```python
from build123d import *
from build123d.topology import SkipClean

# Parameters (mm, degrees)
SKETCH1_W           = 14
SKETCH1_H           = 42
BOSS_EXTRUDE1_DEPTH = 22.5
FILLET1_R           = 2
BOSS_EXTRUDE2_DEPTH = 18.5
BOSS_EXTRUDE3_DEPTH = 5
SKETCH4_R           = 1.1
CUT_EXTRUDE1_DEPTH  = 15
SKETCH5_W           = 2
SKETCH5_H           = 4
BOSS_EXTRUDE4_DEPTH = 5
BOSS_EXTRUDE5_DEPTH = 4
CUT_EXTRUDE2_START  = -2
CUT_EXTRUDE2_DEPTH  = 2
SKETCH12_R          = 3.5
SKETCH12_R_2        = 3.070336519
BOSS_EXTRUDE6_DEPTH = 1
SKETCH14_R          = 3
BOSS_EXTRUDE7_DEPTH = 1
SKETCH15_R          = 1
BOSS_EXTRUDE8_DEPTH = 7
SKETCH16_R          = 2
BOSS_EXTRUDE9_DEPTH = 1.5
CUT_EXTRUDE3_DEPTH  = 18.5


with BuildPart() as part:
    # Sketch1 → Boss-Extrude1 (new body)
    with BuildSketch(Plane(origin=(0, 0, 0), x_dir=(1, 0, 0), z_dir=(0, 1, 0))):
        with Locations((-14.72963025, -0.456790856)):
            Rectangle(SKETCH1_W, SKETCH1_H)
    extrude(amount=BOSS_EXTRUDE1_DEPTH)

    # Fillet1
    fillet1_edges = [part.edges().sort_by_distance(p)[0] for p in [
        (-14.72963025, 22.5, -20.543209144),
        (-14.72963025, 0, -20.543209144),
        (-14.72963025, 0, 21.456790856),
        (-14.72963025, 22.5, 21.456790856),
    ]]
    fillet(fillet1_edges, radius=FILLET1_R)

    # Sketch2 → Boss-Extrude2 (add)
    with BuildSketch(Plane(origin=(-7.72963025, 0, 0), x_dir=(0, 0, -1), z_dir=(1, 0, 0))):
        with BuildLine():
            Line((3.666133326, 18.67433994), (3.666133326, 3.82566006))
            ThreePointArc((3.666133326, 3.82566006), (12.136760187, 0.056811401), (20.543209144, 3.966716207))
            Line((20.543209144, 3.966716207), (20.543209144, 18.533283793))
            ThreePointArc((20.543209144, 18.533283793), (12.136760187, 22.443188599), (3.666133326, 18.67433994))
        make_face()
    extrude(amount=BOSS_EXTRUDE2_DEPTH)

    # Sketch3 → Boss-Extrude3 (add)
    with BuildSketch(Plane(origin=(-7.72963025, 0, 0), x_dir=(0, 0, -1), z_dir=(1, 0, 0))):
        with BuildLine():
            Line((3.666133326, 12.265446457), (3.666133326, 10.341158941))
            ThreePointArc((3.666133326, 10.341158941), (3.170141933, 10.546427574), (2.72390333, 10.248075799))
            ThreePointArc((2.72390333, 10.248075799), (-1.152649836, 11.204898318), (2.678489822, 12.329861741))
            ThreePointArc((2.678489822, 12.329861741), (3.155102255, 12.033793242), (3.666133326, 12.265446457))
        make_face()
    extrude(amount=BOSS_EXTRUDE3_DEPTH)

    # Sketch4 → Cut-Extrude1 (cut)
    with BuildSketch(Plane(origin=(-7.72963025, 0, 0), x_dir=(0, 0, -1), z_dir=(1, 0, 0))):
        with Locations((-18.956790856, 20)):
            Circle(SKETCH4_R)
        with Locations((-18.956790856, 2.5)):
            Circle(SKETCH4_R)
    extrude(amount=-CUT_EXTRUDE1_DEPTH, mode=Mode.SUBTRACT)

    # Sketch5 → Boss-Extrude4 (add)
    with BuildSketch(Plane(origin=(0, 0, -20.543209144), x_dir=(-1, 0, 0), z_dir=(0, 0, -1))):
        with Locations((7.72963025, 11.25)):
            Rectangle(SKETCH5_W, SKETCH5_H)
    extrude(amount=BOSS_EXTRUDE4_DEPTH)

    # Sketch6 → Boss-Extrude5 (add)
    with BuildSketch(Plane(origin=(-6.72963025, 0, 0), x_dir=(0, 0, -1), z_dir=(1, 0, 0))):
        with BuildLine():
            ThreePointArc((21.679339079, 11.975250565), (21.032871281, 11.616126027), (20.543209144, 12.17031195))
            Line((20.543209144, 12.17031195), (20.543209144, 10.774749435))
            ThreePointArc((20.543209144, 10.774749435), (21.198638933, 11.046780591), (21.679339079, 10.524749435))
            ThreePointArc((21.679339079, 10.524749435), (25.543209144, 11.25), (21.679339079, 11.975250565))
        make_face()
    extrude(amount=BOSS_EXTRUDE5_DEPTH)

    # Sketch7 → Cut-Extrude2 (cut)
    with BuildSketch(Plane(origin=(-6.72963025, 0, 0), x_dir=(0, 0, -1), z_dir=(1, 0, 0)).offset(CUT_EXTRUDE2_START)):
        with BuildLine():
            Line((23.543209144, 13.25), (23.543209144, 13.967200788))
            Line((23.543209144, 13.967200788), (25.760178749, 13.967200788))
            Line((25.760178749, 13.967200788), (25.760178749, 8.970470958))
            Line((25.760178749, 8.970470958), (23.543209144, 8.970470958))
            Line((23.543209144, 8.970470958), (23.543209144, 9.25))
            ThreePointArc((23.543209144, 9.25), (25.543209144, 11.25), (23.543209144, 13.25))
        make_face()
    extrude(amount=CUT_EXTRUDE2_DEPTH, mode=Mode.SUBTRACT)

    # Sketch12 → Boss-Extrude6 (add)
    with BuildSketch(Plane.ZY.offset(21.72963025)):
        with Locations(Location((10.456790856, 11.25, 0), (0, 0, 180))):
            Circle(SKETCH12_R)
        with Locations((10.456790856, 11.25)):
            Circle(SKETCH12_R_2, mode=Mode.SUBTRACT)
    extrude(amount=BOSS_EXTRUDE6_DEPTH)

    # Sketch14 → Boss-Extrude7 (add)
    with BuildSketch(Plane.ZY.offset(21.72963025)):
        with Locations(Location((10.456790856, 11.25, 0), (0, 0, 180))):
            Circle(SKETCH14_R)
    extrude(amount=BOSS_EXTRUDE7_DEPTH)

    # Sketch15 → Boss-Extrude8 (add)
    with SkipClean():  # the faces are left unmerged after this step: merging them gives an invalid solid
        with BuildSketch(Plane.ZY.offset(22.72963025)):
            with BuildLine():
                Line((8.853884636, 8.714119157), (8.853884636, 13.785880843))
                ThreePointArc((8.853884636, 13.785880843), (10.456790856, 14.25), (12.059697077, 13.785880843))
                Line((12.059697077, 13.785880843), (12.059697077, 8.714119157))
                ThreePointArc((12.059697077, 8.714119157), (10.456790856, 8.25), (8.853884636, 8.714119157))
            make_face()
            with Locations((10.456790856, 11.25)):
                Circle(SKETCH15_R, mode=Mode.SUBTRACT)
        extrude(amount=BOSS_EXTRUDE8_DEPTH)

    # Sketch16 → Boss-Extrude9 (add)
    with SkipClean():  # the faces are left unmerged after this step: merging them gives an invalid solid
        with BuildSketch(Plane.ZY.offset(21.72963025)):
            with Locations(Location((-0.543209144, 11.25, 0), (0, 0, 180))):
                Circle(SKETCH16_R)
        extrude(amount=BOSS_EXTRUDE9_DEPTH)

    # Sketch17 → Cut-Extrude3 (cut)
    with SkipClean():  # the faces are left unmerged after this step: merging them gives an invalid solid
        with BuildSketch(Plane(origin=(10.77036975, 0, 0), x_dir=(0, 0, -1), z_dir=(1, 0, 0))):
            with BuildLine():
                Line((19.843209144, 4.230369564), (19.843209144, 18.269630436))
                ThreePointArc((19.843209144, 18.269630436), (12.134214683, 21.743184905), (4.366133326, 18.403860381))
                Line((4.366133326, 18.403860381), (4.366133326, 4.096139619))
                ThreePointArc((4.366133326, 4.096139619), (12.134214683, 0.756815095), (19.843209144, 4.230369564))
            make_face()
        extrude(amount=-CUT_EXTRUDE3_DEPTH, mode=Mode.SUBTRACT)


solid = part.part
```
Input: part model. Units: mm. Frame: model coordinates. A direction names the side the tool comes from. Coordinates: 2 decimals unless noted, no trailing zeros. Write each loop counter-clockwise with the first axis right and the second up, starting at its lowest first coordinate (ties: lowest second). Pieces come first, ordered by that corner, then holes.
1) Section B-B on y = 7. Output: boundary loops of the cut face in (x, z), and give its area (3 significant figures).
2) Mould query, pull axis Y, two halves, no side actions, for faces 1 (the flat face through (-7.73, 11, -12)), 2 (the flat face through (-8, 13.25, -22)), 3 (the flat face through (-2.73, 11, -24)). Classes: pulls with the +Y half, pulls with the -Y half, needs draft (parallel to the pull), parting line crosses it, or undercut.
3) Section D-D on x = -26.5. Output: boundary loops of the cut face in (y, z), and give its area (3 significant figures).
4) Section C-C on x = -19. Output: boundary loops of the cut face in (y, z), and give its area (3 significant figures).
5) Pin query (flat end, axial travel): pin 1 Ø1 at (y, z) = (11.5, 10.5) entering from -X; pin 2 Ø3.5 at (y, z) = (11, -1.5) entering from +X; pin 3 Ø9 at (x, y) = (2.5, 7.5) entering from -Z. Return the tip coordinate at first contact, or that it passes through.
6) Set-up query: faces 4 (the flat face through (-22.73, 11, 8)), 5 (the cylindrical face through (-26.181, 10.642, 9.663)), 6 (the cylindrical face through (-4.758, 11.614, -21.044)), 7 (the flat face through (-8, 9.25, -22)), 8 (the flat face through (-8.73, 11, -23)). Return all of +Z, -Z, +X, -X, +Y, -Y with unobstructed straight access to the full face (end or side cutting, diameter ignored); none if empty.
7) Section A-A on x = 2. Output: boundary loops of the cut face in (y, z).
8) Material intervals for line 1 along Z through (x, y) = (-5.5, 8); line 2 along X through (y, z) = (18.5, 3.5); line 3 along X through (y, z) = (13, -21.5), sorted ascending.
Check result:
1. outline: (-21.73, -20.54) - (10.77, -20.54) - (10.77, -19.84) - (-7.73, -19.84) - (-7.73, -4.37) - (10.77, -4.37) - (10.77, -3.67) - (-7.73, -3.67) - (-7.73, 21.46) - (-21.73, 21.46) - close
1. area: 614 mm2
2. face 1: undercut
2. face 2: pulls with the +Y half
2. face 3: needs draft
3. outline: (8.71, 8.85) - (13.79, 8.85) arc R3 ccw to (13.79, 12.06) - (8.71, 12.06) arc R3 ccw to start; hole circle Ø2 at (11.25, 10.46)
3. area: 15.1 mm2
4. outline: (0, -18.54) arc R2 ccw to (2, -20.54) - (20.5, -20.54) arc R2 ccw to (22.5, -18.54) - (22.5, 19.46) arc R2 ccw to (20.5, 21.46) - (2, 21.46) arc R2 ccw to (0, 19.46) - close; hole circle Ø2.2 at (2.5, 18.96); hole circle Ø2.2 at (20, 18.96)
4. area: 934 mm2
5. pin 1: stops at x = -22.73
5. pin 2: stops at x = -2.73
5. pin 3: stops at z = -20.54
6. face 4: -X, +Y, -Y
6. face 5: -X
6. face 6: +X, +Y
6. face 7: -Z, +X, -X, -Y
6. face 8: -Z, -X, +Y, -Y
7. outline: (3.83, -3.67) arc R11.19 ccw to (3.97, -20.54) - (18.53, -20.54) arc R11.19 ccw to (18.67, -3.67) - close; hole (4.1, -4.37) arc R10.49 ccw to (4.23, -19.84) - (18.27, -19.84) arc R10.49 ccw to (18.4, -4.37) - close
8. line 1: z = -20.54 to -19.84, -4.37 to -3.67
8. line 2: x = -21.73 to -7.73
8. line 3: x = -8.73 to -6.73
